Read the model definition and answer for the solid it produces. Units are mm, in the model's axes. Round coordinates to 2 decimals unless told otherwise and drop trailing zeros. Order: outer loops, then holes, each group sorted by start corner. A loop starts at its lowest first (then second) coordinate and runs counter-clockwise, first axis right, second up. Notation, with made-up numbers: (-6, 21.5) - (39, 21.5) arc R13 cw to (39, 44.5) - close; hole circle Ø4 at (31.5, 64). An arc over 180 degrees is marked (long way). Put each result on its own line as item: value. Start each with the question number.
Q1. Section C-C on z = 1.9 is taken. Give the vertices of the cut face in (x, y), then the cut area to 3 significant figures.
Q2. For a pull along Y with two mould halves and no side action, classify faces 1 (the face through (85, 17.018, 2)), 2 (the face through (17.019, 64, 2)), 3 (the face through (-3.307, 106.986, 2.535)), 4 (the face through (70, -18, 2)) as pulls with the +Y half, pulls with the -Y half, needs draft (parallel to the pull), parting line crosses it, or undercut.
Q3. Section D-D on y = 79 is taken. Give the vertices of the cut face in (x, z), then the cut area to 3 significant figures.
Q4. Find the intervals of material crossed by line 1 along Y through (x, z) = (-13, 2.4); line 2 along X through (y, z) = (37.5, 0.9), in increasing order. Write a range as from..to.
Q5. Section B-B on x = -13 is taken. Give the vertices of the cut face in (y, z), then the cut area to 3 significant figures.
Q6. Section A-A on y = -13 is taken. Give the vertices of the cut face in (x, z), then the cut area to 3 significant figures.
from build123d import *

# Parameters (mm, degrees)
BOSS_EXTRUDE1_DEPTH = 5
SKETCH3_R           = 2.5
CUT_EXTRUDE1_DEPTH  = 6


with BuildPart() as part:
    # Sketch2 → Boss-Extrude1 (new body)
    with BuildSketch(Plane.XY):
        Polygon((-18.000000008, 109.507702779), (17.018717612, 109.507702779), (17.018717612, 17.017935082), (155, 17.017935082), (155, -18), (-18.000000008, -18), align=None)
    extrude(amount=BOSS_EXTRUDE1_DEPTH)

    # Sketch3 → Cut-Extrude1 (cut, through all)
    with BuildSketch(Plane.XY.offset(5)):
        with Locations((-13.000000008, -13)):
            Circle(SKETCH3_R)
        with Locations((-2.981282388, 104.507702779)):
            Circle(SKETCH3_R)
    extrude(amount=-CUT_EXTRUDE1_DEPTH, mode=Mode.SUBTRACT)


solid = part.part
Findings:
1. outline: (-18, -18) - (155, -18) - (155, 17.02) - (17.02, 17.02) - (17.02, 109.51) - (-18, 109.51) - close; hole circle Ø5 at (-13, -13); hole circle Ø5 at (-2.98, 104.51)
1. area: 9,260 mm2
2. face 1: pulls with the +Y half
2. face 2: needs draft
2. face 3: undercut
2. face 4: pulls with the -Y half
3. outline: (-18, 0) - (17.02, 0) - (17.02, 5) - (-18, 5) - close
3. area: 175 mm2
4. line 1: -18..-15.5, -10.5..109.51
4. line 2: -18..17.02
5. outline: (-18, 0) - (-15.5, 0) - (-15.5, 5) - (-18, 5) - close; (-10.5, 0) - (109.51, 0) - (109.51, 5) - (-10.5, 5) - close
5. area: 613 mm2
6. outline: (-18, 0) - (-15.5, 0) - (-15.5, 5) - (-18, 5) - close; (-10.5, 0) - (155, 0) - (155, 5) - (-10.5, 5) - close
6. area: 840 mm2
